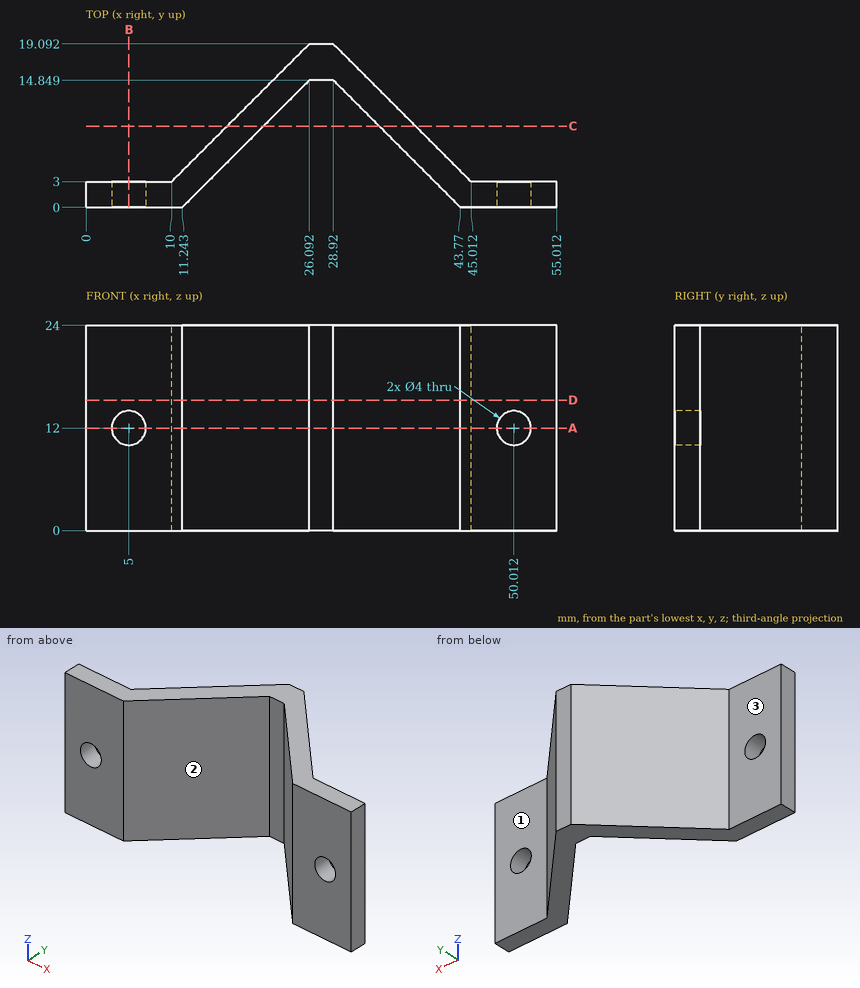
Geometry: see drawing. Coordinates: mm, zero at the bounding-box minimum. A direction names the side the tool comes from. Give positions to 0.01 mm unless a question says otherwise; leave off trailing zeros. Loops run counter-clockwise (first coordinate to the right, second up) from the corner with the lowest first, then second, coordinate; pieces in that order, holes last. Notation, with made-up numbers: (-4.5, 51) -> (51.5, 51) arc R16 cw to (51.5, 72) -> close; hole circle Ø3 at (-15, 43.5). An arc over 180 degrees is marked (long way). Answer as a JSON object with one key per item and string values. Group by question number.
Item 1: Cut plane B-B, the plane x = 5. Return the cut outline in (y, z).
Item 2: Cut plane C-C, the plane y = 9.5. Return the cut outline in (x, z), and give its area (3 significant figures).
Item 3: Cut plane A-A, the plane z = 12. Return the cut outline in (x, y), and give its area (3 significant figures).
Item 4: Line query: probe 1 along X at (y, z) = (0.75, 12) (1 decimal); probe 2 along X at (y, z) = (1.3, 12) (1 decimal); probe 3 along Y at (x, z) = (8, 5.5). Output: solid intervals per line, ascending.
Item 5: Reachability of the marked faces 1, 2 and 3 from +Z, -Z, +X, -X, +Y, -Y: full face, straight path, thin tool, end or side. Return the list, or none.
Item 6: Pin query (flat end, axial travel): P1, Ø6, axis at y = 14, z = 5, coming from the -X side; P2, Ø1, axis at x = 29.5, z = 13.5, coming from the -Y side; P3, Ø3, axis at x = 6, z = 7.5, coming from the +Y side. Return the tip coordinate at first contact, or that it passes through.
Item 7: Cut plane D-D, the plane z = 15.25. Return the cut outline in (x, y).
Checks:
{
 "1": {"outline": "(0, 0) -> (3, 0) -> (3, 10) -> (0, 10) -> close; (0, 14) -> (3, 14) -> (3, 24) -> (0, 24) -> close"},
 "2": {"outline": "(16.5, 0) -> (20.74, 0) -> (20.74, 24) -> (16.5, 24) -> close; (34.27, 0) -> (38.51, 0) -> (38.51, 24) -> (34.27, 24) -> close", "area": "204 mm²"},
 "3": {"outline": "(0, 0) -> (3, 0) -> (3, 3) -> (0, 3) -> close; (7, 0) -> (11.24, 0) -> (26.09, 14.85) -> (28.92, 14.85) -> (43.77, 0) -> (48.01, 0) -> (48.01, 3) -> (45.01, 3) -> (28.92, 19.09) -> (26.09, 19.09) -> (10, 3) -> (7, 3) -> close; (52.01, 0) -> (55.01, 0) -> (55.01, 3) -> (52.01, 3) -> close", "area": "183 mm²"},
 "4": {"probe 1": "x = 0 to 3, 7 to 12, 43 to 48, 52 to 55", "probe 2": "x = 0 to 3, 7 to 12.5, 42.5 to 48, 52 to 55", "probe 3": "y = 0 to 3"},
 "5": {"face 1": "+Z, -Z, +X, +Y", "face 2": "+Z, -Z, -Y", "face 3": "+Z, -Z, -X, +Y"},
 "6": {"P1": "stops at x = 18", "P2": "stops at y = 13.77", "P3": "stops at y = 3"},
 "7": {"outline": "(0, 0) -> (11.24, 0) -> (26.09, 14.85) -> (28.92, 14.85) -> (43.77, 0) -> (55.01, 0) -> (55.01, 3) -> (45.01, 3) -> (28.92, 19.09) -> (26.09, 19.09) -> (10, 3) -> (0, 3) -> close"}
}
